Design review of the part shown in the three views and the two pictorial views. Dimensions are in mm from the part's minimum x, y and z. Round coordinates to 2 decimals unless told otherwise and drop trailing zeros. Loops run counter-clockwise (first coordinate to the right, second up) from the corner with the lowest first, then second, coordinate; pieces in that order, holes last. Notation, with made-up numbers: (51.5, 82) -> (84.5, 82) arc R26 cw to (84.5, 100) -> close; hole circle Ø6 at (-34.5, -12.5). An arc over 180 degrees is marked (long way). Write each question's results on one line, items separated by ' | '. Start each with the question number.
Item 1: We need section A-A (x = 31.75). Give the boundary of the cut face in (y, z), and give its area (4 significant figures).
Item 2: We need section B-B (z = 25.4). Give the boundary of the cut face in (x, y), and give its area (3 significant figures).
Item 3: For L1, parallel to X at y = 5, z = 25.4; L2, parallel to Z at x = 31.75, y = 3; L3, parallel to X at y = 4.5, z = 24, list the stretches that pass through material, from the lowest coordinate up. Write a range as from..to.
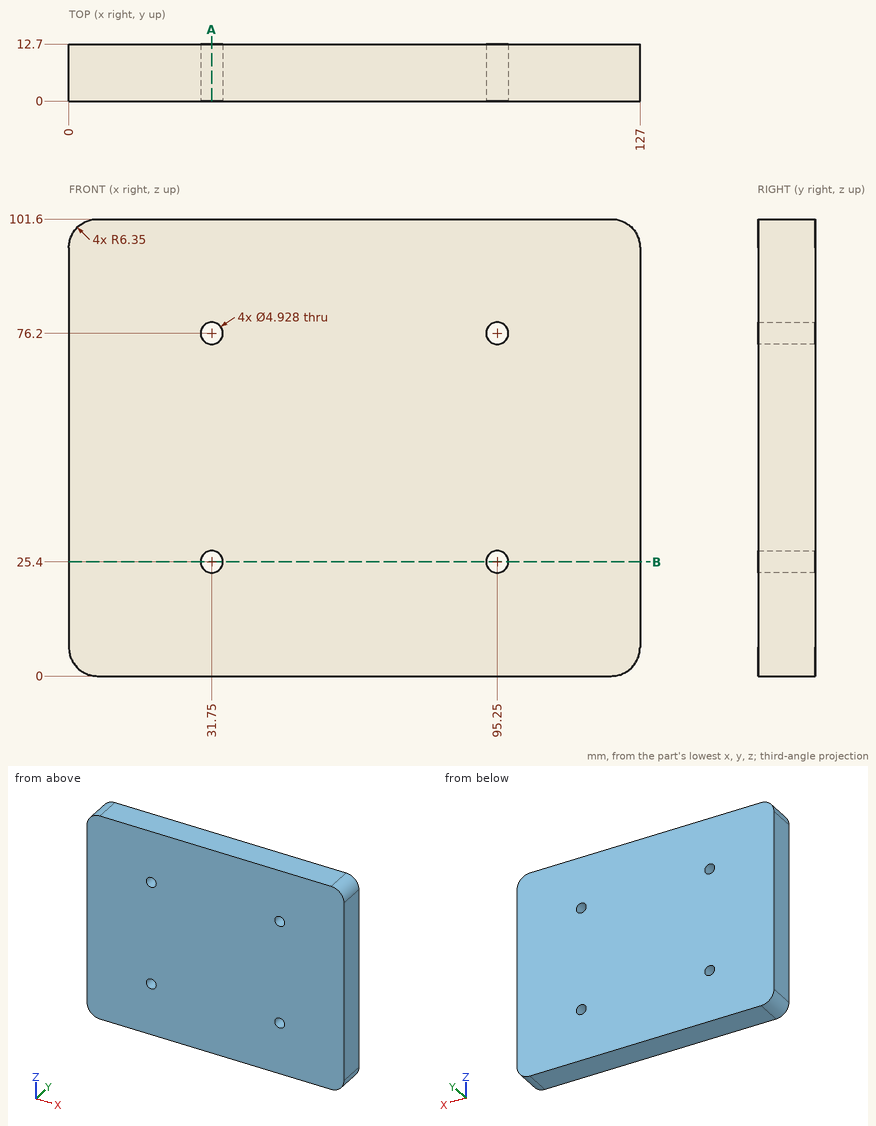
Here are the results:
1) outline: (0, 0) -> (12.7, 0) -> (12.7, 22.94) -> (0, 22.94) -> close; (0, 27.86) -> (12.7, 27.86) -> (12.7, 73.74) -> (0, 73.74) -> close; (0, 78.66) -> (12.7, 78.66) -> (12.7, 101.6) -> (0, 101.6) -> close | area: 1,165 mm2
2) outline: (0, 0) -> (29.29, 0) -> (29.29, 12.7) -> (0, 12.7) -> close; (34.21, 0) -> (92.79, 0) -> (92.79, 12.7) -> (34.21, 12.7) -> close; (97.71, 0) -> (127, 0) -> (127, 12.7) -> (97.71, 12.7) -> close | area: 1,490 mm2
3) L1: x = 0..29.29, 34.21..92.79, 97.71..127 | L2: z = 0..22.94, 27.86..73.74, 78.66..101.6 | L3: x = 0..29.72, 33.78..93.22, 97.28..127
